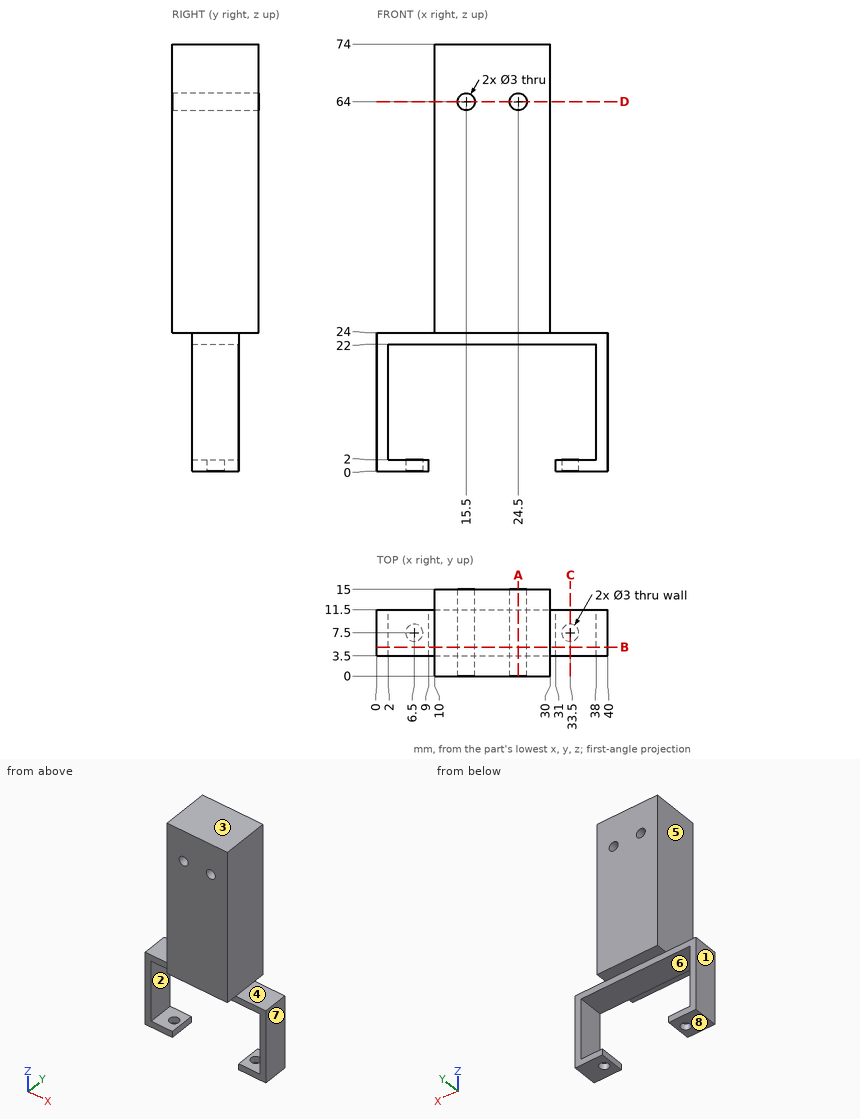
Input: dimensioned drawing with shaded views. Units: mm. Origin: part minimum x, y, z. A direction names the side the tool comes from. Coordinates: 2 decimals unless noted, no trailing zeros. Loops run counter-clockwise (first coordinate to the right, second up) from the corner with the lowest first, then second, coordinate; pieces in that order, holes last. Notation, with made-up numbers: (4, 47) -> (23, 47) arc R25 cw to (23, 67) -> close; hole circle Ø8 at (54.25, 51). An arc over 180 degrees is marked (long way). One line per item, written item: value. Start each with the question number.
Q1. Section query D-D, the plane z = 64. Return the cut outline in (x, y), and give its area (3 significant figures).
Q2. Mould query, pull axis X, two halves, no side actions, for the marked faces 6, 7 and 8. Classes: pulls with the +X half, pulls with the -X half, needs draft (parallel to the pull), parting line crosses it, or undercut.
Q3. Section query A-A, the plane x = 24.5. Return the cut outline in (y, z), and give its area (3 significant figures).
Q4. Section query C-C, the plane x = 33.5. Return the cut outline in (y, z), and give its area (3 significant figures).
Q5. Set-up query: the marked faces 1, 2, 3, 4 and 5. Return all of +Z, -Z, +X, -X, +Y, -Y with unobstructed straight access to the full face (end or side cutting, diameter ignored); none if empty.
Q6. Contact query for flat-ended pins moving along their axis: P1, Ø2.5, axis at x = 33.5, y = 7.5, coming from the -Z side; P2, Ø4, axis at x = 17.5, y = 14, coming from the -Z side; P3, Ø3.5, axis at x = 35, y = 7.5, coming from the +Z side. Output: stop coordinate, or through.
Q7. Section query B-B, the plane y = 5. Return the cut outline in (x, z).
Q8. Line query: line 1 along X through (y, z) = (8.75, 64); line 2 along Y through (x, z) = (33.5, 0.8); line 3 along Z through (x, y) = (6.5, 9.5). Output: solid intervals per line, ascending.
Results:
1. outline: (10, 0) -> (14, 0) -> (14, 15) -> (10, 15) -> close; (17, 0) -> (23, 0) -> (23, 15) -> (17, 15) -> close; (26, 0) -> (30, 0) -> (30, 15) -> (26, 15) -> close
1. area: 210 mm^2
2. face 6: undercut
2. face 7: pulls with the +X half
2. face 8: needs draft
3. outline: (0, 24) -> (3.5, 24) -> (3.5, 22) -> (11.5, 22) -> (11.5, 24) -> (15, 24) -> (15, 62.5) -> (0, 62.5) -> close; (0, 65.5) -> (15, 65.5) -> (15, 74) -> (0, 74) -> close
3. area: 721 mm^2
4. outline: (3.5, 0) -> (6, 0) -> (6, 2) -> (3.5, 2) -> close; (3.5, 22) -> (11.5, 22) -> (11.5, 24) -> (3.5, 24) -> close; (9, 0) -> (11.5, 0) -> (11.5, 2) -> (9, 2) -> close
4. area: 26.0 mm^2
5. face 1: +Z, -Z, -X, +Y, -Y
5. face 2: +Y, -Y
5. face 3: +Z, +X, -X, +Y, -Y
5. face 4: +Z, +X, +Y, -Y
5. face 5: +Z, -X, +Y, -Y
6. P1: z = 22
6. P2: z = 24
6. P3: z = 24
7. outline: (0, 0) -> (9, 0) -> (9, 2) -> (2, 2) -> (2, 22) -> (38, 22) -> (38, 2) -> (31, 2) -> (31, 0) -> (40, 0) -> (40, 24) -> (30, 24) -> (30, 74) -> (10, 74) -> (10, 24) -> (0, 24) -> close; hole circle Ø3 at (15.5, 64); hole circle Ø3 at (24.5, 64)
8. line 1: 10 to 14, 17 to 23, 26 to 30
8. line 2: 3.5 to 6, 9 to 11.5
8. line 3: 0 to 2, 22 to 24
